The listing builds one solid part. Answer for the finished solid, in the listing's coordinates (mm). A direction names the side the tool comes from. Round coordinates to 2 decimals unless told otherwise and drop trailing zeros. Write each loop counter-clockwise with the first axis right and the second up, starting at its lowest first coordinate (ties: lowest second). Pieces come first, ordered by that corner, then holes.
Item 1: Find section B-B on y = 0.75. Give the vertices of the cut face in (x, z).
Item 2: Find section A-A on z = -4.75. Give the vertices of the cut face in (x, y).
Item 3: Find section D-D on y = 4. Give the vertices of the cut face in (x, z).
Item 4: Find section C-C on x = 2.31. Give the vertices of the cut face in (y, z), then the cut area to 3 significant figures.
Item 5: For a pull along X with two mould halves and no side action, classify faces 5 (the face through (5.35, 3, 0)), 6 (the face through (-4.61, 3, 5)), 7 (the face through (1.07, 3.13, 4.59)) as +X half, -X half, draft (parallel to the pull), parting line (faces both ways), or undercut.
Item 6: A tool of negligible diameter and unlimited length cuts with its end or side. For faces 1 (the face through (-6, 4.5, -3)), 2 (the face through (-6, 3, -4.05)), 3 (the face through (-6, 3, -2.02)), 4 (the face through (-6, 1.05, -3)), from which of +Z, -Z, +X, -X, +Y, -Y can it reach the whole face along a straight path? Write none if from no direction.
Item 7: Find the intervals of material crossed by probe 1 along Z at (x, y) = (2.31, 3.25); probe 2 along X at (y, z) = (1.75, -4.75); probe 3 along X at (y, z) = (3.25, 4.75), in increasing order.
Item 8: Each of these flat-tipped pins is pushed along its axis until it touches: pin 1 (0.9 mm diameter, centred on x = -5.5, y = 2.5, fed in from +Z); pin 2 (2 mm diameter, centred on y = 4.5, z = 5, fed in from -X). Where does it stop, or does it pass through?
Autodesk Inventor part; units mm, degrees
ref_plane "YZ Plane" through (0, 0, 0) normal (1, 0, 0) x (0, 1, 0)
ref_plane "XZ Plane" through (0, 0, 0) normal (0, 1, 0) x (-1, 0, 0)
ref_plane "XY Plane" through (0, 0, 0) normal (0, 0, 1) x (1, 0, 0)
sketch "Skizze1" plane through (0, 0, 0) normal (0, 1, 0) x (-1, 0, 0)
  line L0 (-5.35, 10.05) -> (5.35, 10.05)
  line L1 (5.35, 10.05) -> (5.35, -10.05)
  line L2 (5.35, -10.05) -> (-5.35, -10.05)
  line L3 (-5.35, -10.05) -> (-5.35, 10.05)
  line L4 (-5.35, 10.05) -> (5.35, -10.05) construction
  line L5 (5.35, 10.05) -> (-5.35, -10.05) construction
  line L6 (4.61, 10.05) -> (4.61, 0.15)
  line L7 (4.61, 0.15) -> (5.35, -0.59)
  point P0 (0, 0)
  dimension "d0" = 10.7
  dimension "d1" = 20.1
  dimension "d2" = 9.96
  dimension "d3" = 9.9
  dimension "d4" = 45
extrude "Extrusion1" add sketch "Skizze1" along normal blind 6.35 contours L0 L6 L7 L1 L2 L3
sketch "Skizze2" plane through (-5.35, 0, -10.05) normal (-1, 0, 0) x (0, 0, 1)
  line L0 (6, 4.5) -> (8.03, 4.5)
  line L1 (8.03, 4.5) -> (8.03, 1.05)
  line L2 (8.03, 1.05) -> (6, 1.05)
  line L3 (6, 1.05) -> (6, 4.5)
  line L4 (0, 0) -> (9.46, 0)
  line L5 (0, 6.35) -> (9.46, 6.35)
  line L6 (0, 0) -> (0, 6.35)
  point P0 (10.05, 0)
  dimension "d7" = 2.03
  dimension "d8" = 3.45
  dimension "d9" = 1.05
  dimension "d10" = 1.85
  dimension "d11" = 6
extrude "Extrusion2" add sketch "Skizze2" along normal blind 1.6
fillet "Rundung1" radius 0.8 2 edges at (-6.95, 2.775, -2.02) (-6.95, 2.775, -4.05)
sketch "Skizze3" plane through (0, 6.35, 0) normal (0, 1, 0) x (1, 0, 0)
  line L0 (-4.61, -0.15) -> (-4.61, -10.05)
  line L1 (5.35, -10.05) -> (5.35, 10.05)
  line L2 (5.35, 10.05) -> (-5.35, 10.05)
  line L3 (-4.61, -10.05) -> (5.35, -10.05)
  point P0 (0, 0)
  point P1 (2.31, -4.75)
  point P2 (2.31, 4.75)
  dimension "d15" = 9.5
  dimension "d16" = 6.92
  dimension "d17" = 3.04
  dimension "d18" = 0
  dimension "d19" = 5.3
  dimension "d20" = 5.3
hole "Bohrung1" at (2.31, 6.35, 4.75) at (2.31, 6.35, -4.75) direction (0, -1, 0) diameter 2.5 end through all
sketch "Skizze4" plane through (-6.95, 0, -10.05) normal (-1, 0, 0) x (0, 0, 1)
  line L0 (6.8, 1.05) -> (6.8, 4.5)
  line L1 (6.8, 1.05) -> (7.23, 1.05)
  line L2 (7.23, 4.5) -> (7.23, 1.05)
  line L3 (7.23, 4.5) -> (6.8, 4.5)
  circle A0 centre (7.015, 2.775) radius 0.1
  point P0 (10.05, 0)
  dimension "d28" = 0.2
  dimension "d29" = 1.725
  dimension "d30" = 1.725
  dimension "d31" = 0.43
  dimension "d32" = 0.215
extrude "Extrusion3" cut sketch "Skizze4" against normal blind 0.2 contours A0
equation "\"d32\" = 0.5 * d31"
properties part number "MicroswitchBig"
Check values:
1. outline: (-5.35, -10.05) - (5.35, -10.05) - (5.35, 10.05) - (-4.61, 10.05) - (-4.61, 0.15) - (-5.35, -0.59) - close; hole circle Ø2.5 at (2.31, -4.75); hole circle Ø2.5 at (2.31, 4.75)
2. outline: (-5.35, 0) - (1.06, 0) - (1.06, 6.35) - (-5.35, 6.35) - close; (3.56, 0) - (5.35, 0) - (5.35, 6.35) - (3.56, 6.35) - close
3. outline: (-6.95, -3.25) arc R0.8 ccw to (-6.15, -4.05) - (-5.35, -4.05) - (-5.35, -10.05) - (5.35, -10.05) - (5.35, 10.05) - (-4.61, 10.05) - (-4.61, 0.15) - (-5.35, -0.59) - (-5.35, -2.02) - (-6.15, -2.02) arc R0.8 ccw to (-6.95, -2.82) - close; hole circle Ø2.5 at (2.31, -4.75); hole circle Ø2.5 at (2.31, 4.75)
4. outline: (0, -10.05) - (6.35, -10.05) - (6.35, -6) - (0, -6) - close; (0, -3.5) - (6.35, -3.5) - (6.35, 3.5) - (0, 3.5) - close; (0, 6) - (6.35, 6) - (6.35, 10.05) - (0, 10.05) - close
4. area: 95.9 mm2
5. face 5: +X half
5. face 6: -X half
5. face 7: undercut
6. face 1: +Z, -Z, -X, +Y
6. face 2: -Z, -X, +Y, -Y
6. face 3: +Z, -X, +Y, -Y
6. face 4: +Z, -Z, -X, -Y
7. probe 1: z = -10.05 to -6, -3.5 to 3.5, 6 to 10.05
7. probe 2: x = -5.35 to 1.06, 3.56 to 5.35
7. probe 3: x = -4.61 to 1.06, 3.56 to 5.35
8. pin 1: stops at z = -0.29
8. pin 2: stops at x = -4.61
